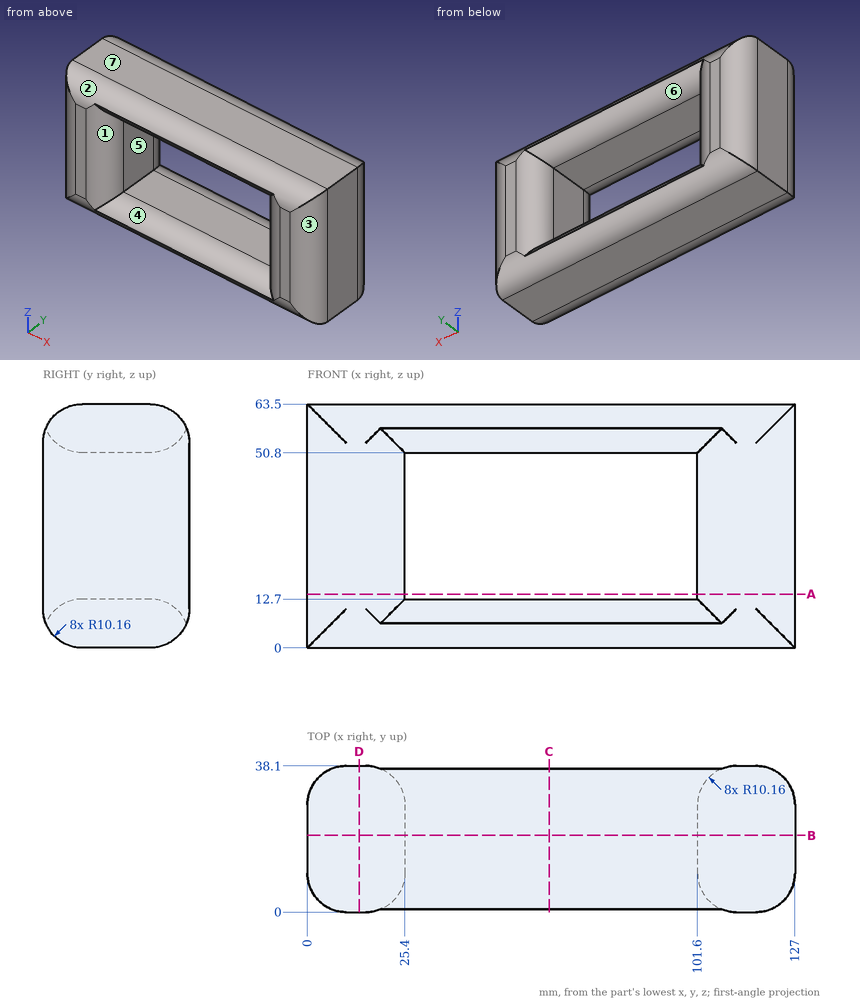
Verification items for this drawing (mm, ordinates from the low corner). A direction names the side the tool comes from. Round coordinates to 2 decimals unless told otherwise and drop trailing zeros. Write each loop counter-clockwise with the first axis right and the second up, starting at its lowest first coordinate (ties: lowest second). Pieces come first, ordered by that corner, then holes. Notation, with made-up numbers: (2.5, 8) - (25.5, 8) arc R30 ccw to (25.5, 41) - close; hole circle Ø10 at (86, 54). An arc over 180 degrees is marked (long way). One line per item, written item: value.
1. Cross-section at A-A on z = 14. Record the boundary of the cut face in (x, y).
The answers:
outline: (0, 10.16) arc R10.16 ccw to (10.16, 0) - (15.24, 0) arc R10.16 ccw to (25.4, 10.16) - (25.4, 27.94) arc R10.16 ccw to (15.24, 38.1) - (10.16, 38.1) arc R10.16 ccw to (0, 27.94) - close; (101.6, 10.16) arc R10.16 ccw to (111.76, 0) - (116.84, 0) arc R10.16 ccw to (127, 10.16) - (127, 27.94) arc R10.16 ccw to (116.84, 38.1) - (111.76, 38.1) arc R10.16 ccw to (101.6, 27.94) - close
2. Cross-section at D-D on x = 13.5. Record the boundary of the cut face in (y, z), and give its area (3 significant figures).
The answers:
outline: (0, 10.16) arc R10.16 ccw to (10.16, 0) - (27.94, 0) arc R10.16 ccw to (38.1, 10.16) - (38.1, 53.34) arc R10.16 ccw to (27.94, 63.5) - (10.16, 63.5) arc R10.16 ccw to (0, 53.34) - close
area: 2,330 mm^2
3. Set-up check for the marked faces 4, 5, 6 and 7: record each of +Z, -Z, +X, -X, +Y, -Y from which the full face is reachable in a straight line by a thin tool's end or side.
The answers:
face 4: -Y
face 5: +Y, -Y
face 6: +Y
face 7: +Z, +X, -X, +Y, -Y
4. Mould release check, pull along Z, two halves, no side actions. Record for the marked faces 1, 2 and 3: released by +Z, released by -Z, zero draft, split by the parting line, or undercut.
The answers:
face 1: undercut
face 2: released by +Z
face 3: zero draft
5. Cross-section at B-B on y = 20. Record the boundary of the cut face in (x, z).
The answers:
outline: (0, 0) - (127, 0) - (127, 63.5) - (0, 63.5) - close; hole (25.4, 12.7) - (101.6, 12.7) - (101.6, 50.8) - (25.4, 50.8) - close
6. Cross-section at C-C on x = 63. Record the boundary of the cut face in (y, z), and give its area (3 significant figures).
The answers:
outline: (0.74, 6.35) arc R10.16 ccw to (10.16, 0) - (27.94, 0) arc R10.16 ccw to (37.36, 6.35) arc R10.16 ccw to (27.94, 12.7) - (10.16, 12.7) arc R10.16 ccw to start; (0.74, 57.15) arc R10.16 ccw to (10.16, 50.8) - (27.94, 50.8) arc R10.16 ccw to (37.36, 57.15) arc R10.16 ccw to (27.94, 63.5) - (10.16, 63.5) arc R10.16 ccw to start
area: 798 mm^2
7. Depth check by flat-ended pin: pin 1 Ø4 at (x, y) = (109, 31.5) entering from -Z; pin 2 Ø10 at (x, z) = (31.5, 13) entering from +Y. Enter the tip coordinate at first touch or a pass-through.
The answers:
pin 1: stops at z = 0.12
pin 2: stops at y = 36.51
8. Scan lines: L1, parallel to Z at x = 76, y = 19.5; L2, parallel to X at y = 24, z = 43; L3, parallel to X at y = 30, z = 45. Record each from-to range of solid material in increasing order.
The answers:
L1: z = 0 to 12.7, 50.8 to 63.5
L2: x = 0 to 25.4, 101.6 to 127
L3: x = 0.21 to 25.19, 101.81 to 126.79
